Read the model definition and answer for the solid it produces. Units are mm, in the model's axes. Coordinates: 2 decimals unless noted, no trailing zeros. Write each loop counter-clockwise with the first axis right and the second up, starting at its lowest first coordinate (ties: lowest second). Pieces come first, ordered by that corner, then holes. Notation, with made-up numbers: M 73.5,-4.5 L 77.5,-4.5 A7 ccw 77.5,3.5 Z; hole C 60.25,76.25 d2. An arc over 180 degrees is marked long. Use a Markdown table: item, result. Add a question column.
from build123d import *

# Parameters (mm, degrees)
SKETCH_1_R      = 1.65
SKETCH_1_R_2    = 2
SKETCH_1_R_3    = 1.6
SKETCH_1_R_4    = 2.1
EXTRUDE_1_DEPTH = 4


with BuildPart() as part:
    # 草图1 → 凸台-拉伸1 (new body)
    with BuildSketch(Plane.XY):
        with BuildLine():
            Line((-115, -5.384342662), (-71.257490086, -5.384342662))
            ThreePointArc((-71.257490086, -5.384342662), (-66.066099293, -6.837444884), (-62.383432799, -10.774450336))
            Line((-62.383432799, -10.774450336), (-60.183484139, -15.009358454))
            ThreePointArc((-60.183484139, -15.009358454), (-57.254551951, -22.080426266), (-50.183484139, -25.009358454))
            Line((-50.183484139, -25.009358454), (-25.933484139, -25.009358454))
            ThreePointArc((-25.933484139, -25.009358454), (-18.862416327, -27.938290642), (-15.933484139, -35.009358454))
            Line((-15.933484139, -35.009358454), (-15.933484139, -63.56099727))
            Line((-15.933484139, -63.56099727), (15.933484139, -63.56099727))
            Line((15.933484139, -63.56099727), (15.933484139, -35.009358454))
            ThreePointArc((15.933484139, -35.009358454), (18.862416327, -27.938290642), (25.933484139, -25.009358454))
            Line((25.933484139, -25.009358454), (50.183484139, -25.009358454))
            ThreePointArc((50.183484139, -25.009358454), (57.254551951, -22.080426266), (60.183484139, -15.009358454))
            Line((60.183484139, -15.009358454), (62.383432799, -10.774450336))
            ThreePointArc((62.383432799, -10.774450336), (66.066099293, -6.837444884), (71.257490086, -5.384342662))
            Line((71.257490086, -5.384342662), (115, -5.384342662))
            ThreePointArc((115, -5.384342662), (122.071067812, -2.455410474), (125, 4.615657338))
            Line((125, 4.615657338), (125, 27.373111507))
            ThreePointArc((125, 27.373111507), (122.559714668, 33.919157194), (116.429857174, 37.270359027))
            Line((116.429857174, 37.270359027), (52.621904203, 46.488705755))
            ThreePointArc((52.621904203, 46.488705755), (48.343394427, 46.950893444), (44.042761161, 47.105220638))
            Line((44.042761161, 47.105220638), (0.159946942, 47.105220638))
            Line((0.159946942, 47.105220638), (-0.159946942, 47.105220638))
            Line((-0.159946942, 47.105220638), (-44.042761161, 47.105220638))
            ThreePointArc((-44.042761161, 47.105220638), (-48.343394427, 46.950893444), (-52.621904203, 46.488705755))
            Line((-52.621904203, 46.488705755), (-116.429857174, 37.270359027))
            ThreePointArc((-116.429857174, 37.270359027), (-122.559714668, 33.919157194), (-125, 27.373111507))
            Line((-125, 27.373111507), (-125, 4.615657338))
            ThreePointArc((-125, 4.615657338), (-122.071067812, -2.455410474), (-115, -5.384342662))
        make_face()
        with Locations((0, -54.709358454)):
            Circle(SKETCH_1_R, mode=Mode.SUBTRACT)
        with Locations((-10.5, -44.209358454)):
            Circle(SKETCH_1_R, mode=Mode.SUBTRACT)
        with Locations((-10.5, -23.209358454)):
            Circle(SKETCH_1_R, mode=Mode.SUBTRACT)
        with Locations((-49, -17.209358454)):
            Circle(SKETCH_1_R, mode=Mode.SUBTRACT)
        with Locations((-25, -12.709358454)):
            Circle(SKETCH_1_R, mode=Mode.SUBTRACT)
        with Locations((10.5, -44.209358454)):
            Circle(SKETCH_1_R, mode=Mode.SUBTRACT)
        with Locations((0, -33.709358454)):
            Circle(SKETCH_1_R, mode=Mode.SUBTRACT)
        with Locations((10.5, -23.209358454)):
            Circle(SKETCH_1_R, mode=Mode.SUBTRACT)
        with Locations((0, -12.709358454)):
            Circle(SKETCH_1_R, mode=Mode.SUBTRACT)
        with Locations((25, -12.709358454)):
            Circle(SKETCH_1_R, mode=Mode.SUBTRACT)
        with Locations((49, -17.209358454)):
            Circle(SKETCH_1_R, mode=Mode.SUBTRACT)
        with Locations((-110, 6.402358032)):
            Circle(SKETCH_1_R_2, mode=Mode.SUBTRACT)
        with Locations((-120.5, 16.902358032)):
            Circle(SKETCH_1_R_2, mode=Mode.SUBTRACT)
        with Locations((-99.5, 16.902358032)):
            Circle(SKETCH_1_R_2, mode=Mode.SUBTRACT)
        with Locations((-0.4, 1.032228913)):
            Circle(SKETCH_1_R_3, mode=Mode.SUBTRACT)
        with Locations((-7.4, 8.032228913)):
            Circle(SKETCH_1_R_3, mode=Mode.SUBTRACT)
        with Locations((-0.4, 15.032228913)):
            Circle(SKETCH_1_R_3, mode=Mode.SUBTRACT)
        with Locations((-110, 27.402358032)):
            Circle(SKETCH_1_R_2, mode=Mode.SUBTRACT)
        with Locations((-0.4, 22.032228913)):
            Circle(SKETCH_1_R_3, mode=Mode.SUBTRACT)
        with Locations((-7.4, 29.032228913)):
            Circle(SKETCH_1_R_3, mode=Mode.SUBTRACT)
        with Locations((-0.4, 36.032228913)):
            Circle(SKETCH_1_R_3, mode=Mode.SUBTRACT)
        with Locations((-0.4, 42.532228913)):
            Circle(SKETCH_1_R_4, mode=Mode.SUBTRACT)
        with Locations((6.6, 8.032228913)):
            Circle(SKETCH_1_R_3, mode=Mode.SUBTRACT)
        with Locations((10.1, 11.532228913)):
            Circle(SKETCH_1_R_3, mode=Mode.SUBTRACT)
        with Locations((3.1, 18.532228913)):
            Circle(SKETCH_1_R_3, mode=Mode.SUBTRACT)
        with Locations((17.1, 18.532228913)):
            Circle(SKETCH_1_R_3, mode=Mode.SUBTRACT)
        with Locations((110, 6.402358032)):
            Circle(SKETCH_1_R_2, mode=Mode.SUBTRACT)
        with Locations((99.5, 16.902358032)):
            Circle(SKETCH_1_R_2, mode=Mode.SUBTRACT)
        with Locations((120.5, 16.902358032)):
            Circle(SKETCH_1_R_2, mode=Mode.SUBTRACT)
        with Locations((10.1, 25.532228913)):
            Circle(SKETCH_1_R_3, mode=Mode.SUBTRACT)
        with Locations((6.6, 29.032228913)):
            Circle(SKETCH_1_R_3, mode=Mode.SUBTRACT)
        with Locations((9.6, 42.532228913)):
            Circle(SKETCH_1_R_4, mode=Mode.SUBTRACT)
        with Locations((110, 27.402358032)):
            Circle(SKETCH_1_R_2, mode=Mode.SUBTRACT)
    extrude(amount=EXTRUDE_1_DEPTH)


solid = part.part
Item 1: Each of these flat-tipped pins is pushed along its axis until it touches: pin 1 (1 mm diameter, centred on x = -98.5, z = 1.5, fed in from -Y); pin 2 (1.5 mm diameter, centred on x = -52, z = 2.5, fed in from +Y); pin 3 (2 mm diameter, centred on x = 34.5, z = 1.5, fed in from -Y). Where does it stop, or does it pass through?
Item 2: Find section C-C on x = 80. Give the vertices of the cut face in (y, z).
Item 3: Find section A-A on x = -35. Give the vertices of the cut face in (y, z), then the cut area to 3 significant figures.
Item 4: Consider probe 1 along Y at (x, z) = (-11.5, 1.8); probe 2 along X at (y, z) = (16, 2.75); probe 3 along Y at (x, z) = (10.1, 2.45). Determine where each line is inside the solid, lowest interval first.
Item 5: Find section B-B on z = 2.8. Count the separate pieces of the cut face and the enclosed holes in it, then the cut area to 3 significant figures.
Item 6: Determine the mould class of faces 1 (the cylindrical face through (9.145, 40.482, 1.972)), 2 (the flat face through (-84.079, 41.944, 1.972)), 3 (the cylindrical face through (66, -6.88, 1.97)) for opening direction X: pulls with the +X half, pulls with the -X half, needs draft (parallel to the pull), parting line crosses it, or undercut.
Geometry says:
| question | item | result |
|---|---|---|
| 1 | pin 1 | stops at y = -5.38 |
| 1 | pin 2 | stops at y = 46.67 |
| 1 | pin 3 | stops at y = -25.01 |
| 2 | outline | M -5.38,0 L 42.53,0 L 42.53,4 L -5.38,4 Z |
| 3 | outline | M -25.01,0 L 47.11,0 L 47.11,4 L -25.01,4 Z |
| 3 | area | 288 mm2 |
| 4 | probe 1 | y = -63.56 to -45.52, -42.9 to -24.52, -21.9 to 47.11 |
| 4 | probe 2 | x = -125 to -122.28, -118.72 to -101.28, -97.72 to -1.67, 0.87 to 97.72, 101.28 to 118.72, 122.28 to 125 |
| 4 | probe 3 | y = -63.56 to -45.81, -42.61 to -24.81, -21.61 to 9.93, 13.13 to 23.93, 27.13 to 40.49, 44.57 to 47.11 |
| 5 | separate pieces | 1 |
| 5 | enclosed holes | 33 |
| 5 | area | 15,500 mm2 |
| 6 | face 1 | undercut |
| 6 | face 2 | pulls with the -X half |
| 6 | face 3 | pulls with the +X half |
